from build123d import *

# Parameters (mm, degrees)
DODANIE_WYCI_GNI_CIE1_DEPTH = 14.2
SZKIC2_W                    = 1.2
SZKIC2_H                    = 10.85
DODANIE_WYCI_GNI_CIE3_DEPTH = 29.25
SZKIC6_W                    = 4.251450278
SZKIC6_H                    = 1.2
DODANIE_WYCI_GNI_CIE4_DEPTH = 3
SZKIC20_R                   = 1.5
WYTNIJ_WYCI_GNI_CIE5_DEPTH  = 10
WYTNIJ_WYCI_GNI_CIE3_DEPTH  = 0.5
SZKIC11_R                   = 0.5
DODANIE_WYCI_GNI_CIE5_DEPTH = 29.25
WYTNIJ_WYCI_GNI_CIE6_DEPTH  = 10
SZKIC23_R                   = 1.5
WYTNIJ_WYCI_GNI_CIE8_DEPTH  = 10


with BuildPart() as part:
    # Szkic1 → Dodanie-wyciągnięcie1 (new body)
    with BuildSketch(Plane.XY):
        Polygon((-36.878659539, 9.21375), (-5.378659539, 9.21375), (-5.378659539, 14.41375), (-22.378659539, 20.06375), (-36.878659539, 20.06375), align=None)
    extrude(amount=DODANIE_WYCI_GNI_CIE1_DEPTH)

    # Szkic2 → Dodanie-wyciągnięcie3 (add)
    with BuildSketch(Plane.ZY.offset(36.878659539)):
        with Locations((7.1, 14.63875)):
            Rectangle(SZKIC2_W, SZKIC2_H)
    extrude(amount=DODANIE_WYCI_GNI_CIE3_DEPTH)

    # Szkic6 → Dodanie-wyciągnięcie4 (add)
    with BuildSketch(Plane(origin=(0, 20.06375, 0), x_dir=(1, 0, 0), z_dir=(0, 1, 0))):
        with Locations((-64.0029344, -7.1)):
            Rectangle(SZKIC6_W, SZKIC6_H)
    extrude(amount=DODANIE_WYCI_GNI_CIE4_DEPTH)

    # Szkic20 → Wytnij-wyciągnięcie5 (cut)
    with BuildSketch(Plane.XY.offset(7.7)):
        with Locations((-40.378659539, 14.63375)):
            Circle(SZKIC20_R)
    extrude(amount=-WYTNIJ_WYCI_GNI_CIE5_DEPTH, mode=Mode.SUBTRACT)

    # Szkic10 → Wytnij-wyciągnięcie3 (cut)
    with BuildSketch(Plane.XZ.offset(-9.21375)):
        Polygon((-33.729246345, 6.369364803), (-33.729246345, 14.2), (-32.729246345, 14.2), (-32.729246345, 0), (-33.729246345, 0), align=None)
    extrude(amount=-WYTNIJ_WYCI_GNI_CIE3_DEPTH, mode=Mode.SUBTRACT)

    # Szkic11 → Dodanie-wyciągnięcie5 (add)
    with BuildSketch(Plane.ZY.offset(36.878659539)):
        with Locations((7.85, 18.36375)):
            Circle(SZKIC11_R)
    extrude(amount=DODANIE_WYCI_GNI_CIE5_DEPTH)

    # Szkic21 → Wytnij-wyciągnięcie6 (cut)
    with BuildSketch(Plane(origin=(0, 0, 6.5), x_dir=(-1, 0, 0), z_dir=(0, 0, -1))):
        Polygon((55.478659539, 9.21375), (66.128659539, 9.21375), (66.128659539, 11.81375), (57.478659539, 11.81375), align=None)
    extrude(amount=-WYTNIJ_WYCI_GNI_CIE6_DEPTH, mode=Mode.SUBTRACT)

    # Szkic23 → Wytnij-wyciągnięcie8 (cut)
    with BuildSketch(Plane(origin=(0, 0, 6.5), x_dir=(-1, 0, 0), z_dir=(0, 0, -1))):
        with Locations((48.378659539, 14.63375)):
            Circle(SZKIC23_R)
    extrude(amount=-WYTNIJ_WYCI_GNI_CIE8_DEPTH, mode=Mode.SUBTRACT)


solid = part.part
Model file for the job. Use its own axes, mm. A direction names the side the tool comes from. Coordinates: 2 decimals unless noted, no trailing zeros. Write each loop counter-clockwise with the first axis right and the second up, starting at its lowest first coordinate (ties: lowest second). Pieces come first, ordered by that corner, then holes. Notation, with made-up numbers: (-22, 23) - (2, 23) arc R6 ccw to (2, 27) - close; hole circle Ø8 at (-18, 41.25). An arc over 180 degrees is marked (long way). Write each question's results on one line, items separated by ' | '. Start each with the question number.
1) Cut at B-B (x = -48). Write the cut outline in (y, z), then the cut area to 3 significant figures.
2) Flat gauge pins, fed straight in: P1, Ø7, axis at x = -48.5, y = 12, coming from the +Z side; P2, Ø1.5, axis at x = -17, y = 20, coming from the +Z side; P3, Ø5, axis at y = 14.5, z = 3.5, coming from the -X side; P4, Ø4, axis at x = -55.5, y = 14.5, coming from the -Z side. Where does each tip first touch, or does it go through?
3) Cut at C-C (x = -58). Write the cut outline in (y, z).
4) Cut at D-D (y = 21.5). Write the cut outline in (x, z), then the cut area to 3 significant figures.
5) Probe line 1 along Y through (x, z) = (-35, 1.5); line 2 along Z through (x, y) = (-41, 20); line 3 along Y through (x, z) = (-56, 8). List the from-to ranges inside material, lowest first. Write a range as from..to.
6) Mould opens along Z. For faces 4 (the face through (-51.3, 18.35, 8.35)), 5 (the face through (-21, 15, 0)), 6 (the face through (-33, 9.714, 7)) say: pulls with the +Z half, pulls with the -Z half, needs draft (parallel to the pull), parting line crosses it, or undercut.
7) 3-axis set-ups, long thin cutter, end or side, ignore diameter. For faces 1 (the face through (-19, 9.214, 7)), 2 (the face through (-52, 15, 6.5)), 3 (the face through (-61.877, 22, 7)): which of +Z, -Z, +X, -X, +Y, -Y reach the whole face in a straight line?
8) Cut at A-A (y = 15.25). Write the cut outline in (x, z), then the cut area to 3 significant figures.
Returned:
1) outline: (9.21, 6.5) - (13.18, 6.5) - (13.18, 7.7) - (9.21, 7.7) - close; (16.09, 6.5) - (20.06, 6.5) - (20.06, 7.7) - (18.84, 7.7) arc R0.5 ccw (long way) to (17.89, 7.7) - (16.09, 7.7) - close | area: 10.1 mm^2
2) P1: z = 7.7 | P2: through | P3: x = -36.88 | P4: z = 6.5
3) outline: (11.81, 6.5) - (20.06, 6.5) - (20.06, 7.7) - (18.84, 7.7) arc R0.5 ccw (long way) to (17.89, 7.7) - (11.81, 7.7) - close
4) outline: (-66.13, 6.5) - (-61.88, 6.5) - (-61.88, 7.7) - (-66.13, 7.7) - close | area: 5.10 mm^2
5) line 1: 9.21..20.06 | line 2: 6.5..7.7 | line 3: 17.89..18.84
6) face 4: undercut | face 5: pulls with the -Z half | face 6: needs draft
7) face 1: +Z, -Z, +X, -X, -Y | face 2: -Z, -X, +Y, -Y | face 3: +Z, -Z, +X, +Y
8) outline: (-66.13, 6.5) - (-49.75, 6.5) - (-49.75, 7.7) - (-66.13, 7.7) - close; (-47.01, 6.5) - (-41.75, 6.5) - (-41.75, 7.7) - (-47.01, 7.7) - close; (-39.01, 6.5) - (-36.88, 6.5) - (-36.88, 0) - (-7.89, 0) - (-7.89, 14.2) - (-36.88, 14.2) - (-36.88, 7.7) - (-39.01, 7.7) - close | area: 440 mm^2
